For this review, use the dimensioned drawing (mm, ordinates from the lowest corner) and the shaded views. A direction names the side the tool comes from. Coordinates: 2 decimals unless noted, no trailing zeros. Loops run counter-clockwise (first coordinate to the right, second up) from the corner with the lowest first, then second, coordinate; pieces in that order, holes last. Notation, with made-up numbers: M 22,63 L 72,63 A4 ccw 72,70 Z; hole C 13,61.5 d7. An arc over 180 degrees is marked long. Write item = value, one per line.
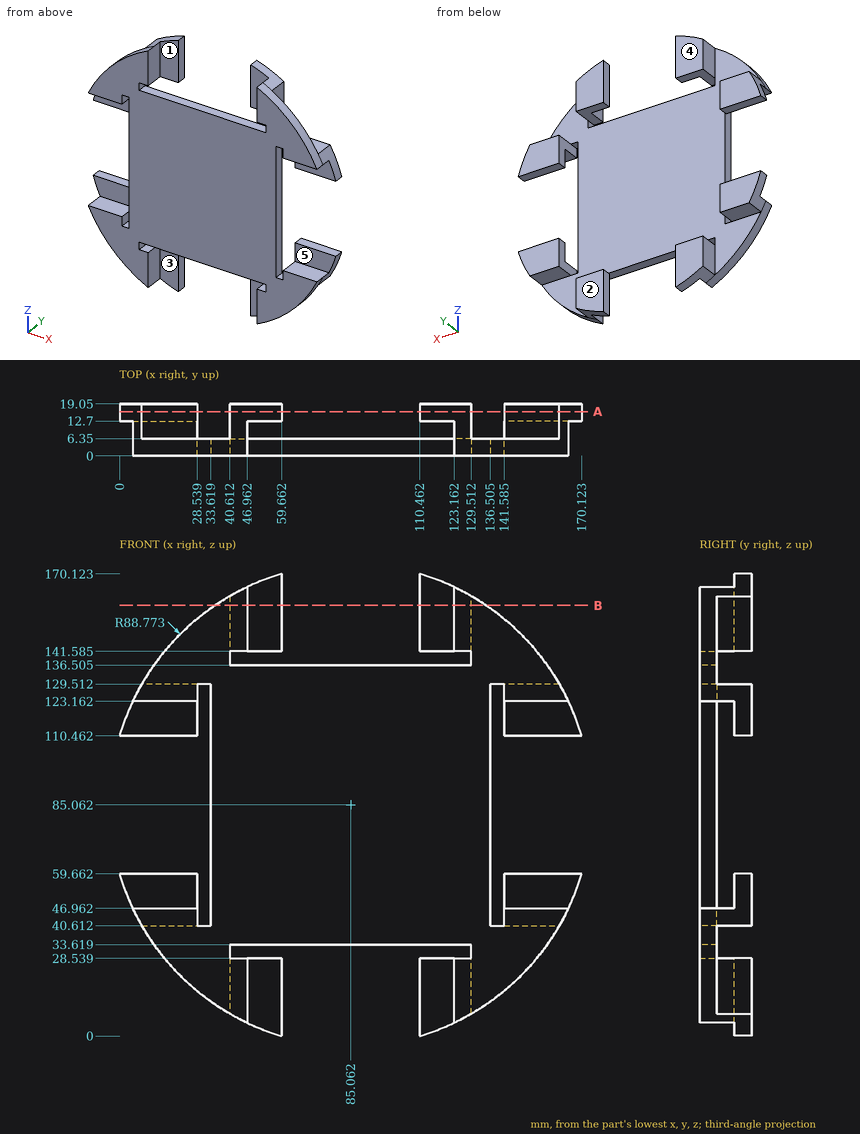
Q1. For line 1 along X through (y, z) = (9.5, 14.5); line 2 along X through (y, z) = (2.25, 143), list the stretches that pass through material, from the lowest coordinate up.
Solved:
line_1 = 40.61 to 46.96, 123.16 to 129.51
line_2 = 17.8 to 46.96, 123.16 to 152.32
Q2. Add section B-B (z = 158.5). Write out the cut boundary in (x, y), and give its area (3 significant figures).
Solved:
outline = M 35.19,0 L 46.96,0 L 46.96,12.7 L 59.66,12.7 L 59.66,19.05 L 40.61,19.05 L 40.61,6.35 L 35.19,6.35 Z; M 110.46,12.7 L 123.16,12.7 L 123.16,0 L 134.94,0 L 134.94,6.35 L 129.51,6.35 L 129.51,19.05 L 110.46,19.05 Z
area = 472 mm²
Q3. For pin 1 Ø2 at (y, z) = (3.5, 65.5) entering from +X (1 decimal); pin 2 Ø10 at (x, y) = (25.5, 7) entering from -Z; pin 3 Ø1.9 at (x, y) = (86.5, 3.5) entering from -Z, all flat-tipped, find the tip position at first contact; note any pin that passes through.
Solved:
pin_1 = 136.5
pin_2 = 15.07
pin_3 = 33.62
Q4. Draft analysis for pull direction X (two halves, no side actions). For the marked faces 1 and 2, state which applies: +X half, -X half, draft (parallel to the pull), parting line (faces both ways), or undercut.
Solved:
face_1 = undercut
face_2 = draft
Q5. Machinability: for the marked faces 3, 4 and 5, which of the approach directions +Z, -Z, +X, -X, +Y, -Y give a long, thin tool a straight path to every point of the face, cutting with its end or side? Answer none if there is none.
Solved:
face_3 = +Z, -Z, -Y
face_4 = +Z, -Z, +X, -X, +Y
face_5 = +X, -X, -Y
Q6. Add section A-A (y = 16.25). State how many separate pieces and enclosed holes the cut face has, and give its area (3 significant figures).
Solved:
separate_pieces = 8
enclosed_holes = 0
area = 3,790 mm²
